Read the model definition and answer for the solid it produces. Units are mm, in the model's axes. Round coordinates to 2 decimals unless told otherwise and drop trailing zeros. Loops run counter-clockwise (first coordinate to the right, second up) from the corner with the lowest first, then second, coordinate; pieces in that order, holes last. Notation, with made-up numbers: (52.25, 53) - (74.25, 53) arc R16 cw to (74.25, 76) - close; hole circle Ø8 at (-5.75, 7.25). An arc over 180 degrees is marked (long way). Answer as CSV lines item,"result".
```python
from build123d import *

# Parameters (mm, degrees)
F0_W      = 46
F0_H      = 22
F1_DEPTH  = 235
F2_R      = 1.5
F3_W      = 3.5
F3_H      = 16
F3_W_2    = 1.5
F4_DEPTH  = 46.001
F5_W      = 16
F5_H      = 5
F6_DEPTH  = 235.001
F7_R      = 4
F8_DEPTH  = 17.001
F9_R      = 7
F9_R_2    = 4
F10_DEPTH = 10


with BuildPart() as f1:
    # F0 (on Top) → F1 (new body)
    with BuildSketch(Plane.XY):
        with Locations((23, 11)):
            Rectangle(F0_W, F0_H)
    extrude(amount=F1_DEPTH)

    # F2
    f2_edges = [f1.edges().sort_by_distance(p)[0] for p in [
        (46, 0, 117.5),
        (46, 22, 117.5),
        (0, 0, 117.5),
        (0, 22, 117.5),
    ]]
    fillet(f2_edges, radius=F2_R)

    # F3 (on face) → F4 (cut, through all)
    with BuildSketch(Plane(origin=(0, 0, 0), x_dir=(0, -1, 0), z_dir=(-1, 0, 0))):
        with Locations((-3.25, 212)):
            Rectangle(F3_W, F3_H)
        with Locations((-0.75, 212)):
            Rectangle(F3_W_2, F3_H)
    extrude(amount=-F4_DEPTH, mode=Mode.SUBTRACT)

    # F5 (on face) → F6 (cut, through all)
    with BuildSketch(Plane.XY.offset(235)):
        with Locations((23, 2.5)):
            Rectangle(F5_W, F5_H)
    extrude(amount=-F6_DEPTH, mode=Mode.SUBTRACT)

    # F7 (on face) → F8 (cut, through all)
    with BuildSketch(Plane.XZ.offset(-5)):
        with Locations((23, 212)):
            Circle(F7_R)
    extrude(amount=-F8_DEPTH, mode=Mode.SUBTRACT)

    # F9 (on face) → F10 (cut)
    with BuildSketch(Plane(origin=(0, 22, 0), x_dir=(-1, 0, 0), z_dir=(0, 1, 0))):
        with Locations((-23, 212)):
            Circle(F9_R)
        with Locations((-23, 212)):
            Circle(F9_R_2, mode=Mode.SUBTRACT)
    extrude(amount=-F10_DEPTH, mode=Mode.SUBTRACT)


solid = f1.part
```
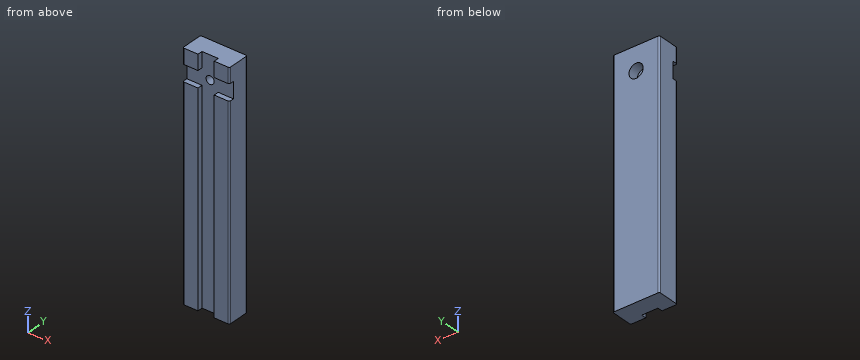
1) A cutting plane is placed at B-B, the plane z = 212. Determine the outline of the cut face in (x, y), plus the area to 3 significant figures.
Entries:
outline,"(0, 5) - (19, 5) - (19, 12) - (16, 12) - (16, 22) - (1.5, 22) arc R1.5 ccw to (0, 20.5) - close; (27, 5) - (46, 5) - (46, 20.5) arc R1.5 ccw to (44.5, 22) - (30, 22) - (30, 12) - (27, 12) - close"
area,"585 mm^2"
2) A cutting plane is placed at A-A, the plane x = 23. Determine the outline of the cut face in (y, z), plus the area to 3 significant figures.
Entries:
outline,"(5, 0) - (22, 0) - (22, 205) - (12, 205) - (12, 208) - (5, 208) - close; (5, 216) - (12, 216) - (12, 219) - (22, 219) - (22, 235) - (5, 235) - close"
area,"3,800 mm^2"
3) Find the intervals of material crossed by line 1 (Z direction, x = 23, y = 9.5); line 2 (X direction, y = 8, z = 212); line 3 (X direction, y = 1.5, z = 36.5), in increasing order.
Entries:
line 1,"z = 0 to 208, 216 to 235"
line 2,"x = 0 to 19, 27 to 46"
line 3,"x = 0 to 15, 31 to 46"
4) A cutting plane is placed at C-C, the plane z = 175.5. Determine the outline of the cut face in (x, y).
Entries:
outline,"(0, 1.5) arc R1.5 ccw to (1.5, 0) - (15, 0) - (15, 5) - (31, 5) - (31, 0) - (44.5, 0) arc R1.5 ccw to (46, 1.5) - (46, 20.5) arc R1.5 ccw to (44.5, 22) - (1.5, 22) arc R1.5 ccw to (0, 20.5) - close"
5) This flat-tipped pin is pushed along its axis until it touches: P1, Ø9, axis at x = 23, z = 212, coming from the -Y side. Where does it stop, or does it pass through?
Entries:
P1,"stops at y = 5"
